Geometry check sheet. Reference: the model listing, model coordinates, mm. Face numbers are marked on the shaded views. Round coordinates to 2 decimals unless told otherwise and drop trailing zeros. Write each loop counter-clockwise with the first axis right and the second up, starting at its lowest first coordinate (ties: lowest second). Pieces come first, ordered by that corner, then holes.
Item 1: Depth check by flat-ended pin: P1, Ø1.5, axis at x = -35.5, y = 12, coming from the +Z side; P2, Ø1, axis at x = 56, z = -21, coming from the -Y side; P3, Ø2, axis at y = 41, z = -59.5, coming from the -X side (3 decimals). Enter the tip coordinate at first touch or a pass-through.
Item 2: Scan lines: probe 1 along X at (y, z) = (47.5, -67); probe 2 along X at (y, z) = (71, -72); probe 3 along Y at (x, z) = (71, -46). Record each from-to range of solid material in increasing order.
Item 3: Draft check along X on the marked faces 1 and 2. Enter one of: pulls with the +X half, pulls with the -X half, needs draft (parallel to the pull), parting line crosses it, or undercut.
Item 4: Cross-section at A-A (x = 22). Enter the section's corners in (y, z), then the cut area to 3 significant figures.
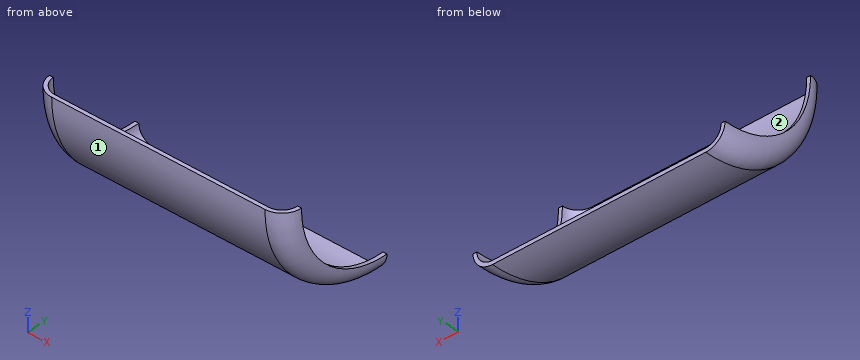
from build123d import *


with BuildPart() as part:
    # Sweep1: sweep along a path in Sketch2
    with BuildLine(Plane(origin=(0, 0, 0), x_dir=(0, 0, -1), z_dir=(1, 0, 0))) as sweep1_path:
        ThreePointArc((0, 0), (53.881536726, 22.318463274), (76.2, 76.2))
    # Sketch1 → Sweep1 (sweep)
    with BuildSketch(Plane.XY):
        with BuildLine():
            Line((-69.85, 0), (69.85, 0))
            ThreePointArc((69.85, 0), (78.830256121, 3.719743879), (82.55, 12.7))
            Line((82.55, 12.7), (80.01, 12.7))
            ThreePointArc((80.01, 12.7), (77.034204897, 5.515795103), (69.85, 2.54))
            Line((69.85, 2.54), (-69.85, 2.54))
            ThreePointArc((-69.85, 2.54), (-77.034204897, 5.515795103), (-80.01, 12.7))
            Line((-80.01, 12.7), (-82.55, 12.7))
            ThreePointArc((-82.55, 12.7), (-78.830256121, 3.719743879), (-69.85, 0))
        make_face()
    sweep(path=sweep1_path.line)


solid = part.part
Resolved:
1. P1: stops at z = -34.75
1. P2: stops at y = 2.81
1. P3: stops at x = -81.675
2. probe 1: x = -78.4 to -73.73, 73.73 to 78.4
2. probe 2: x = -79.11 to -75.12, 75.12 to 79.11
2. probe 3: y = 15.52 to 18.75
3. face 1: needs draft
3. face 2: undercut
4. outline: (0, 0) arc R76.2 ccw to (76.2, -76.2) - (76.2, -73.66) arc R73.66 cw to (2.54, 0) - close
4. area: 299 mm2
